Geometry: see drawing. Coordinates: mm, zero at the bounding-box minimum. A direction names the side the tool comes from. Round coordinates to 2 decimals unless told otherwise and drop trailing zeros. Loops run counter-clockwise (first coordinate to the right, second up) from the corner with the lowest first, then second, coordinate; pieces in that order, holes last.
(1) Set-up query: the marked faces 1, 2 and 3. Return all of +Z, -Z, +X, -X, +Y, -Y with unobstructed straight access to the full face (end or side cutting, diameter ignored); none if empty.
(2) Section B-B, the plane z = 22.5. Return the cut outline in (x, y), plus the area to 3 significant figures.
(3) Section C-C, the plane y = 7.5. Return the cut outline in (x, z), plus the area to 3 significant figures.
(4) Section A-A, the plane x = 26.5. Return the cut outline in (y, z), plus the area to 3 significant figures.
(5) First-contact query: pin 1 Ø5 at (x, y) = (27, 5) entering from +Z; pin 2 Ø4 at (x, z) = (11.5, 30.5) entering from -Y; pin 3 Ø8 at (x, y) = (24.5, 3) entering from -Z. Flat tips, straight axial feed; report the tip coordinate or a pass-through.
(6) Material intervals for probe 1 along Y at (x, z) = (46, 14); probe 2 along X at (y, z) = (6, 19), sorted ascending.
(7) Section D-D, the plane z = 34. Return the cut outline in (x, y).
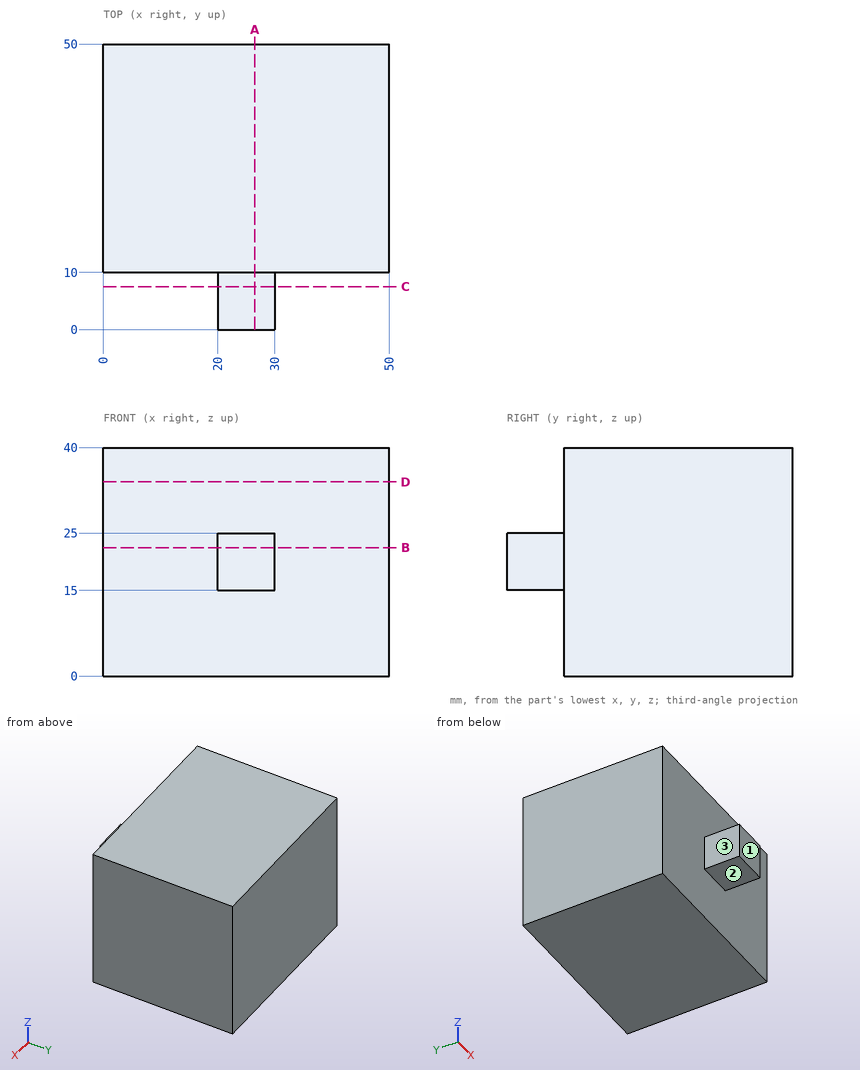
Output values:
1. face 1: +Z, -Z, +X, -X, -Y
1. face 2: -Z, +X, -X, -Y
1. face 3: +Z, -Z, -X, -Y
2. outline: (0, 10) - (20, 10) - (20, 0) - (30, 0) - (30, 10) - (50, 10) - (50, 50) - (0, 50) - close
2. area: 2,100 mm2
3. outline: (20, 15) - (30, 15) - (30, 25) - (20, 25) - close
3. area: 100 mm2
4. outline: (0, 15) - (10, 15) - (10, 0) - (50, 0) - (50, 40) - (10, 40) - (10, 25) - (0, 25) - close
4. area: 1,700 mm2
5. pin 1: stops at z = 25
5. pin 2: stops at y = 10
5. pin 3: stops at z = 15
6. probe 1: y = 10 to 50
6. probe 2: x = 20 to 30
7. outline: (0, 10) - (50, 10) - (50, 50) - (0, 50) - close
